For this review, take the finished solid that the model builds, in its own axes (mm). Coordinates: 2 decimals unless noted, no trailing zeros. Loops run counter-clockwise (first coordinate to the right, second up) from the corner with the lowest first, then second, coordinate; pieces in that order, holes last. Notation, with made-up numbers: (-6.75, 72) - (44.25, 72) arc R7 ccw to (44.25, 79) - close; hole circle Ø1 at (3.25, 22.5). An arc over 180 degrees is marked (long way). Use one line per item in the form item = value. Start each with the question number.
1. For pin 1 Ø0.8 at (x, z) = (-1.5, 1.5) entering from +Y; pin 2 Ø0.8 at (y, z) = (-1, 1) entering from +X; pin 3 Ø1.2 at (x, z) = (0, 1) entering from -Y, all flat-tipped, find the tip position at first contact; note any pin that passes through.
2. Add section D-D on x = -14. Give the boundary of the cut face in (y, z), and give its area (3 significant figures).
3. To check wall thickness, follow probe 1 along Y at (x, z) = (23, 1.55); probe 2 along Y at (x, z) = (15, 1.3); probe 3 along X at (y, z) = (-18, 1.1). State the ranges of each line that lie inside material, in increasing order.
4. Add section C-C on y = -22. Give the boundary of the cut face in (x, z).
5. Add section A-A on x = 0. Give the boundary of the cut face in (y, z), and give its area (3 significant figures).
6. Add section B-B on z = 0.7. Count the separate pieces of the cut face and the enclosed holes in it, and give its area (3 significant figures).
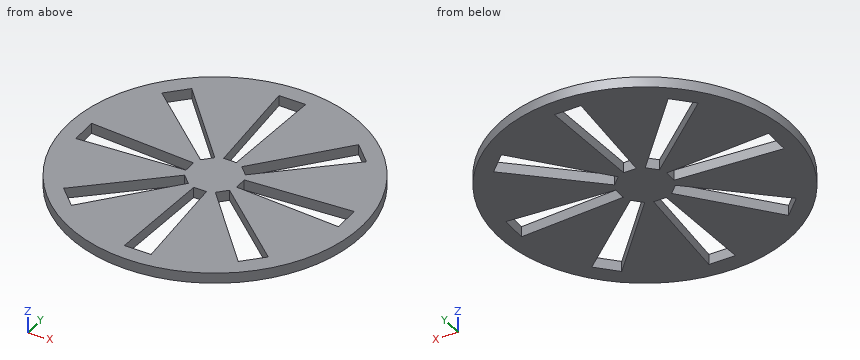
```python
from build123d import *

# Parameters (mm, degrees)
SKETCH1_R           = 35
BOSS_EXTRUDE1_DEPTH = 2.5


with BuildPart() as part:
    # Sketch1 → Boss-Extrude1 (new body)
    with BuildSketch(Plane.XY):
        Circle(SKETCH1_R)
        Polygon((3.15, 31), (-3.15, 31), (-1.5, 6), (1.5, 6), align=None, mode=Mode.SUBTRACT)
        Polygon((19.692923856, 24.147696578), (3.181980515, 5.303300859), (5.303300859, 3.181980515), (24.147696578, 19.692923856), align=None, mode=Mode.SUBTRACT)
        Polygon((31, 3.15), (6, 1.5), (6, -1.5), (31, -3.15), align=None, mode=Mode.SUBTRACT)
        Polygon((24.147696578, -19.692923856), (5.303300859, -3.181980515), (3.181980515, -5.303300859), (19.692923856, -24.147696578), align=None, mode=Mode.SUBTRACT)
        Polygon((3.15, -31), (1.5, -6), (-1.5, -6), (-3.15, -31), align=None, mode=Mode.SUBTRACT)
        Polygon((-19.692923856, -24.147696578), (-3.181980515, -5.303300859), (-5.303300859, -3.181980515), (-24.147696578, -19.692923856), align=None, mode=Mode.SUBTRACT)
        Polygon((-31, -3.15), (-6, -1.5), (-6, 1.5), (-31, 3.15), align=None, mode=Mode.SUBTRACT)
        Polygon((-24.147696578, 19.692923856), (-5.303300859, 3.181980515), (-3.181980515, 5.303300859), (-19.692923856, 24.147696578), align=None, mode=Mode.SUBTRACT)
    extrude(amount=BOSS_EXTRUDE1_DEPTH)


solid = part.part
```
Conclusion:
q1.pin_1 = 34.98
q1.pin_2 = 34.99
q1.pin_3 = -35
q2.outline = (-32.08, 0) - (-17.65, 0) - (-17.65, 2.5) - (-32.08, 2.5) - close; (-10.8, 0) - (-2.03, 0) - (-2.03, 2.5) - (-10.8, 2.5) - close; (2.03, 0) - (10.8, 0) - (10.8, 2.5) - (2.03, 2.5) - close; (17.65, 0) - (32.08, 0) - (32.08, 2.5) - (17.65, 2.5) - close
q2.area = 116 mm^2
q3.probe_1 = -26.38 to -20.84, -18.69 to -2.62, 2.62 to 18.69, 20.84 to 26.38
q3.probe_2 = -31.62 to -18.79, -11.68 to -2.09, 2.09 to 11.68, 18.79 to 31.62
q3.probe_3 = -30.02 to -22.22, -14.31 to -2.29, 2.29 to 14.31, 22.22 to 30.02
q4.outline = (-27.22, 0) - (-21.84, 0) - (-21.84, 2.5) - (-27.22, 2.5) - close; (-17.81, 0) - (-2.56, 0) - (-2.56, 2.5) - (-17.81, 2.5) - close; (2.56, 0) - (17.81, 0) - (17.81, 2.5) - (2.56, 2.5) - close; (21.84, 0) - (27.22, 0) - (27.22, 2.5) - (21.84, 2.5) - close
q5.outline = (-35, 0) - (-31, 0) - (-31, 2.5) - (-35, 2.5) - close; (-6, 0) - (6, 0) - (6, 2.5) - (-6, 2.5) - close; (31, 0) - (35, 0) - (35, 2.5) - (31, 2.5) - close
q5.area = 50.0 mm^2
q6.separate_pieces = 1
q6.enclosed_holes = 8
q6.area = 2,920 mm^2
